Here's how the part is built. I have some questions about the finished solid (model axes, mm). Face numbers are marked on the shaded views. A direction names the side the tool comes from. Coordinates: 2 decimals unless noted, no trailing zeros. Write each loop counter-clockwise with the first axis right and the second up, starting at its lowest first coordinate (ties: lowest second). Pieces come first, ordered by that corner, then holes. Notation, with made-up numbers: (-29, 11) -> (-8, 11) arc R15 ccw to (-8, 18) -> close; hole circle Ø8 at (87.25, -36). An arc over 180 degrees is marked (long way). Use a Markdown table: item, result. Add a question column.
Item 1: Imagine slicing it at C-C, the plane y = -0.5. Write out the boundary of the cut face in (x, z), and give its area (3 significant figures).
Item 2: Imagine slicing it at B-B, the plane x = 17.17. Write out the boundary of the cut face in (y, z) (3 decimals).
Item 3: On a 3-axis mill with a long thin cutter (end or side, diameter ignored), from which of +Z, -Z, +X, -X, +Y, -Y can I reach the whole of each face in a straight line? I mean the marked faces 1, 2, 3, 4 and 5. Say none if no direction works.
Item 4: If I drill on line 1 along X through (y, z) = (2, -0.3); line 2 along X through (y, z) = (7.25, -0.5); line 3 along X through (y, z) = (-4, -1.2), over which ranges is the centre line in solid material (lowest first)? Write a range as from..to.
Item 5: Imagine slicing it at A-A, the plane z = -1.3. Write out the boundary of the cut face in (x, y) (3 decimals), and give its area (3 significant figures).
Item 6: Imagine slicing it at D-D, the plane x = 3. Write out the boundary of the cut face in (y, z) (3 decimals).
Item 7: Will these pins go through, and if not, where does the flat tip stop? pin 1 Ø8 at (x, y) = (-16.5, 1.5) entering from -Z; pin 2 Ø1.6 at (x, z) = (1.5, -1) entering from -Y (3 decimals); pin 3 Ø1 at (x, z) = (1, -1) entering from +Y (3 decimals); pin 4 Ø1 at (x, z) = (-12, -1) entering from +Y (3 decimals).
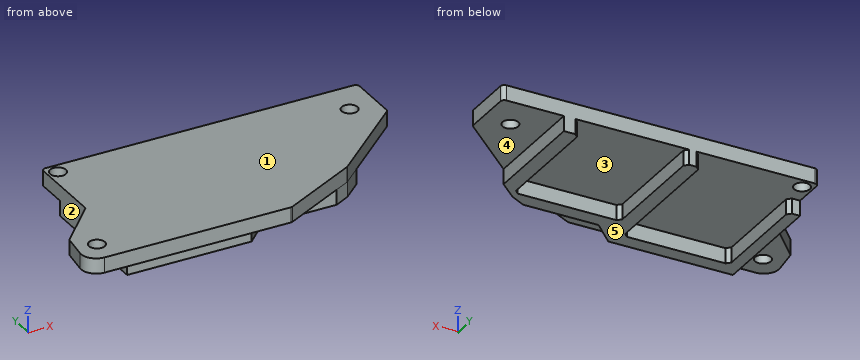
```python
from build123d import *

# Parameters (mm, degrees)
ESQUISSE1_R        = 1.05
BOSS_EXTRU_1_DEPTH = 2
CONG_1_R           = 2
CONG_2_R           = 0.5
BOSS_EXTRU_2_DEPTH = 2
CHANFREIN1_SIZE    = 0.5


with BuildPart() as part:
    # Esquisse1 → Boss.-Extru.1 (new body)
    with BuildSketch(Plane.XY):
        Polygon((-20.8, 10.895), (20.8, 10.895), (20.8, 3.765359203), (10.324093605, -5.633066028), (0.127924824, -10.895), (-20.8, -10.895), (-26.825567122, -10.895), (-26.065636187, -5.293625083), (-20.8, 0.415783742), align=None)
        with Locations((17.17, 6.195)):
            Circle(ESQUISSE1_R, mode=Mode.SUBTRACT)
        with Locations((-19.43, 9.435)):
            Circle(ESQUISSE1_R, mode=Mode.SUBTRACT)
        with Locations((-23.770918846, -7.705)):
            Circle(ESQUISSE1_R, mode=Mode.SUBTRACT)
    extrude(amount=BOSS_EXTRU_1_DEPTH)

    # Congé1
    cong_1_edges = [part.edges().sort_by_distance(p)[0] for p in [
        (-26.825567122, -10.895, 1),
    ]]
    fillet(cong_1_edges, radius=CONG_1_R)

    # Congé2
    cong_2_edges = [part.edges().sort_by_distance(p)[0] for p in [
        (-20.8, 10.895, 1),
        (20.8, 10.895, 1),
        (20.8, 3.765359203, 1),
        (10.324093605, -5.633066028, 1),
        (0.127924824, -10.895, 1),
    ]]
    fillet(cong_2_edges, radius=CONG_2_R)

    # Esquisse2 → Boss.-Extru.2 (add)
    with BuildSketch(Plane(origin=(0, 0, 0), x_dir=(-1, 0, 0), z_dir=(0, 0, -1))):
        Polygon((-10.723313352, 9.373462564), (-10.723313352, -4.635), (3.276686648, -4.635), (3.276686648, 9.365), (3.276686648, 10.895), (5.226686648, 10.895), (5.226686648, 6.495), (5.226686648, -7.505), (19.226686648, -7.505), (19.226686648, 6.495), (20.8, 6.495), (20.8, -9.505), (4.398259523, -9.505), (1.528259523, -6.635), (-8.382623427, -6.635), (-10.371769863, -5.590293429), (-12.723313352, -3.480613862), (-12.723313352, 10.895), (-10.723313352, 10.895), align=None)
    extrude(amount=BOSS_EXTRU_2_DEPTH)

    # Chanfrein1
    chanfrein1_edges = [part.edges().sort_by_distance(p)[0] for p in [
        (10.723313352, 10.895, -1),
        (-19.226686648, 6.495, -1),
        (-19.226686648, -7.505, -1),
        (-5.226686648, -7.505, -1),
        (-5.226686648, 10.895, -1),
        (-3.276686648, 10.895, -1),
        (-3.276686648, -4.635, -1),
        (10.723313352, -4.635, -1),
    ]]
    chamfer(chanfrein1_edges, length=CHANFREIN1_SIZE)


solid = part.part
```
Ans:
| question | item | result |
|---|---|---|
| 1 | outline | (-21.64, 0) -> (-20.8, 0) -> (-20.8, -2) -> (-19.23, -2) -> (-19.23, 0) -> (-5.23, 0) -> (-5.23, -2) -> (-3.28, -2) -> (-3.28, 0) -> (10.72, 0) -> (10.72, -2) -> (12.72, -2) -> (12.72, 0) -> (16.05, 0) -> (16.05, 2) -> (-21.64, 2) -> close |
| 1 | area | 86.4 mm^2 |
| 2 | outline | (0.509, 0) -> (5.145, 0) -> (5.145, 2) -> (0.509, 2) -> close; (7.245, 0) -> (10.895, 0) -> (10.895, 2) -> (7.245, 2) -> close |
| 3 | face 1 | +Z, +X, -X, +Y, -Y |
| 3 | face 2 | -Z, -X, +Y |
| 3 | face 3 | -Z, +Y |
| 3 | face 4 | -Z, +X, +Y, -Y |
| 3 | face 5 | -Z, +X, -X, +Y, -Y |
| 4 | line 1 | x = -20.8..-19.23, -5.23..-3.28, 10.72..12.72 |
| 4 | line 2 | x = -5.23..-3.28, 10.72..12.72 |
| 4 | line 3 | x = -20.8..-19.23, -5.23..-3.28, 10.72..12.14 |
| 5 | outline | (-20.8, -9.505) -> (-4.398, -9.505) -> (-1.528, -6.635) -> (8.383, -6.635) -> (10.372, -5.59) -> (12.723, -3.481) -> (12.723, 10.895) -> (11.223, 10.895) -> (10.723, 10.395) -> (10.723, -4.135) -> (10.223, -4.635) -> (-2.777, -4.635) -> (-3.277, -4.135) -> (-3.277, 10.395) -> (-3.777, 10.895) -> (-4.727, 10.895) -> (-5.227, 10.395) -> (-5.227, -7.005) -> (-5.727, -7.505) -> (-18.727, -7.505) -> (-19.227, -7.005) -> (-19.227, 5.995) -> (-19.727, 6.495) -> (-20.8, 6.495) -> close |
| 5 | area | 151 mm^2 |
| 6 | outline | (-9.413, 0) -> (-6.635, 0) -> (-6.635, -2) -> (-4.635, -2) -> (-4.635, 0) -> (10.895, 0) -> (10.895, 2) -> (-9.413, 2) -> close |
| 7 | pin 1 | stops at z = -2 |
| 7 | pin 2 | stops at y = -6.635 |
| 7 | pin 3 | stops at y = -4.635 |
| 7 | pin 4 | stops at y = -7.505 |
